The model under review builds one solid part; all positions refer to its coordinate system, in mm. A direction names the side the tool comes from. Give positions to 0.01 mm unless a question says otherwise; leave off trailing zeros. Write each loop counter-clockwise with the first axis right and the second up, starting at its lowest first coordinate (ties: lowest second). Pieces come first, ordered by that corner, then holes.
from build123d import *

# Parameters (mm, degrees)
BOSS_EXTRUDE1_DEPTH = 12.7
CUT_EXTRUDE1_DEPTH  = 3.175
SKETCH3_R           = 2.8575
CUT_EXTRUDE2_DEPTH  = 25.4
SKETCH4_R           = 3.571875
CUT_EXTRUDE4_DEPTH  = 2.54
CHAMFER1_SIZE       = 0.79375


with BuildPart() as part:
    # Sketch1 → Boss-Extrude1 (new body)
    with BuildSketch(Plane.XY):
        with BuildLine():
            Line((71.4375, -19.3675), (71.4375, 19.3675))
            ThreePointArc((71.4375, 19.3675), (69.205653673, 24.755653673), (63.8175, 26.9875))
            Line((63.8175, 26.9875), (-63.8175, 26.9875))
            ThreePointArc((-63.8175, 26.9875), (-69.205653673, 24.755653673), (-71.4375, 19.3675))
            Line((-71.4375, 19.3675), (-71.4375, -19.3675))
            ThreePointArc((-71.4375, -19.3675), (-69.205653673, -24.755653673), (-63.8175, -26.9875))
            Line((-63.8175, -26.9875), (63.8175, -26.9875))
            ThreePointArc((63.8175, -26.9875), (69.205653673, -24.755653673), (71.4375, -19.3675))
        make_face()
    extrude(amount=-BOSS_EXTRUDE1_DEPTH)

    # Sketch2 → Cut-Extrude1 (cut)
    with BuildSketch(Plane.XY):
        with BuildLine():
            Line((68.4625, -17.4625), (68.4625, 17.4625))
            ThreePointArc((68.4625, 17.4625), (66.544049417, 22.094049417), (61.9125, 24.0125))
            Line((61.9125, 24.0125), (-61.9125, 24.0125))
            ThreePointArc((-61.9125, 24.0125), (-66.544049417, 22.094049417), (-68.4625, 17.4625))
            Line((-68.4625, 17.4625), (-68.4625, -17.4625))
            ThreePointArc((-68.4625, -17.4625), (-66.544049417, -22.094049417), (-61.9125, -24.0125))
            Line((-61.9125, -24.0125), (61.9125, -24.0125))
            ThreePointArc((61.9125, -24.0125), (66.544049417, -22.094049417), (68.4625, -17.4625))
        make_face()
    extrude(amount=-CUT_EXTRUDE1_DEPTH, mode=Mode.SUBTRACT)

    # Sketch3 → Cut-Extrude2 (cut)
    with BuildSketch(Plane.XZ.offset(26.9875)):
        with Locations((0, -6.35)):
            Circle(SKETCH3_R)
    extrude(amount=-CUT_EXTRUDE2_DEPTH, mode=Mode.SUBTRACT)

    # Sketch4 → Cut-Extrude4 (cut)
    with BuildSketch(Plane.XZ.offset(26.9875)):
        with Locations((0, -6.35)):
            Circle(SKETCH4_R)
    extrude(amount=-CUT_EXTRUDE4_DEPTH, mode=Mode.SUBTRACT)

    # Chamfer1
    chamfer1_edges = [part.edges().sort_by_distance(p)[0] for p in [
        (0, -26.9875, 0),
        (-69.205653673, -24.755653673, 0),
        (-71.4375, 0, 0),
        (-69.205653673, 24.755653673, 0),
        (-69.205653673, -24.755653673, -12.7),
        (0, -26.9875, -12.7),
        (69.205653673, -24.755653673, -12.7),
        (71.4375, 0, -12.7),
        (69.205653673, 24.755653673, -12.7),
        (0, 26.9875, -12.7),
        (-69.205653673, 24.755653673, -12.7),
        (0, 26.9875, 0),
        (-71.4375, 0, -12.7),
        (69.205653673, 24.755653673, 0),
        (71.4375, 0, 0),
        (69.205653673, -24.755653673, 0),
    ]]
    chamfer(chamfer1_edges, length=CHAMFER1_SIZE)


solid = part.part
1) To check wall thickness, follow probe 1 along Z at (x, y) = (0, -25); probe 2 along Z at (x, y) = (0, -18.5) (1 decimal); probe 3 along Y at (x, z) = (62, -1.25). State the ranges of each line that lie inside material, in increasing order.
2) Consider section C-C, the plane y = 8. Give the boundary of the cut face in (x, z) (1 decimal), then the cut area to 3 significant figures.
3) Consider section D-D, the plane x = 0. Give the boundary of the cut face in (y, z) (1 decimal), then the cut area to 3 significant figures.
4) Consider section B-B, the plane z = -6.35. Give the boundary of the cut face in (x, y), then the cut area to 3 significant figures.
5) Insertion check: pin 1 (2 mm diameter, centred on x = 1.5, z = -7, fed in from -Y); pin 2 (2 mm diameter, centred on x = 41, y = 5.5, fed in from +Z) (3 decimals). Each pin has a flat end and moves straight along its axis. Give the tip position at first contact, or say it passes through.
6) Consider section A-A, the plane x = -29. Give the boundary of the cut face in (y, z) (1 decimal), then the cut area to 3 significant figures.
7) Tool access review of faces 4 (the cylindrical face through (-66.595, -22.043, -1.565)), 5 (the cylindrical face through (-0.62, -13.18, -9.14)), 6 (the flat face through (0, -25, 0)): name each direction out of +Z, -Z, +X, -X, +Y, -Y from which nothing blocks a thin tool from reaching the whole face with its end or side.
8) The part is to be moulded in two halves that separate along X. For faces 1 (the flat face through (-68.462, 0, -2)), 2 (the cylindrical face through (-69.15, 24.81, -6.27)), 3 (the flat face through (71.438, 0, -6)), say which applies: +X half, -X half, draft (parallel to the pull), parting line (faces both ways), or undercut.
Answer block:
1. probe 1: z = -12.7 to -9.92, -2.78 to 0
1. probe 2: z = -12.7 to -9.2, -3.5 to -3.2
1. probe 3: y = -26.99 to -24.01, 24.01 to 26.99
2. outline: (-71.4, -11.9) - (-70.6, -12.7) - (70.6, -12.7) - (71.4, -11.9) - (71.4, -0.8) - (70.6, 0) - (68.5, 0) - (68.5, -3.2) - (-68.5, -3.2) - (-68.5, 0) - (-70.6, 0) - (-71.4, -0.8) - close
2. area: 1,380 mm2
3. outline: (-27, -11.9) - (-26.2, -12.7) - (26.2, -12.7) - (27, -11.9) - (27, -0.8) - (26.2, 0) - (24, 0) - (24, -3.2) - (-24, -3.2) - (-24, 0) - (-26.2, 0) - (-27, -0.8) - (-27, -2.8) - (-24.4, -2.8) - (-24.4, -3.5) - (-1.6, -3.5) - (-1.6, -9.2) - (-24.4, -9.2) - (-24.4, -9.9) - (-27, -9.9) - close
3. area: 383 mm2
4. outline: (-71.44, -19.37) arc R7.62 ccw to (-63.82, -26.99) - (-3.57, -26.99) - (-3.57, -24.45) - (-2.86, -24.45) - (-2.86, -1.59) - (2.86, -1.59) - (2.86, -24.45) - (3.57, -24.45) - (3.57, -26.99) - (63.82, -26.99) arc R7.62 ccw to (71.44, -19.37) - (71.44, 19.37) arc R7.62 ccw to (63.82, 26.99) - (-63.82, 26.99) arc R7.62 ccw to (-71.44, 19.37) - close
4. area: 7,510 mm2
5. pin 1: stops at y = -1.59
5. pin 2: stops at z = -3.175
6. outline: (-27, -11.9) - (-26.2, -12.7) - (26.2, -12.7) - (27, -11.9) - (27, -0.8) - (26.2, 0) - (24, 0) - (24, -3.2) - (-24, -3.2) - (-24, 0) - (-26.2, 0) - (-27, -0.8) - close
6. area: 532 mm2
7. face 4: +Z
7. face 5: -Y
7. face 6: +Z, +X, -X, +Y, -Y
8. face 1: undercut
8. face 2: -X half
8. face 3: +X half
